Source: CAD feature listing. Evaluate the final solid. Frame: model axes, mm. Face numbers are marked on the shaded views. Coordinates: 2 decimals unless noted, no trailing zeros. Loops run counter-clockwise (first coordinate to the right, second up) from the corner with the lowest first, then second, coordinate; pieces in that order, holes last. Notation, with made-up numbers: M 2.25,3.25 L 20.25,3.25 A26 cw 20.25,42.25 Z; hole C -33,-2 d6. An arc over 180 degrees is marked long. One line per question, with ' | ' between items. Start each with the question number.
1. Mould query, pull axis Z, two halves, no side actions, for the marked faces 1, 2, 3 and 4. Classes: pulls with the +Z half, pulls with the -Z half, needs draft (parallel to the pull), parting line crosses it, or undercut.
2. Ray query, probe 1 along Y at (x, z) = (0, 0); probe 2 along Y at (x, z) = (0, 5.5); probe 3 along Z at (x, y) = (1.75, 0). Return the intervals inside material, ascending.
3. Pin query (flat end, axial travel): P1, Ø2, axis at x = 4.5, z = -0.5, coming from the -Y side; P2, Ø3, axis at y = 0, z = 0, coming from the +X side. Return the tip coordinate at first contact, or that it passes through.
4. Section query B-B, the plane z = 0. Output: boundary loops of the cut face in (x, y), and give its area (3 significant figures).
5. Section query A-A, the plane x = 0. Output: boundary loops of the cut face in (y, z), and give its area (3 significant figures).
6. Section query C-C, the plane y = -14. Output: boundary loops of the cut face in (x, z), and give its area (3 significant figures).
7. Section query D-D, the plane x = 4.75. Output: boundary loops of the cut face in (y, z), and give its area (3 significant figures).
```python
from build123d import *

# Parameters (mm, degrees)
SKETCH_R          = 1.6
PAD_DEPTH         = 6
SKETCH001_R       = 1.6
POCKET_DEPTH      = 6.001
POCKET_DEPTH_BACK = -6.001
FILLET_R          = 3


with BuildPart() as part:
    # Sketch → Pad (new body, symmetric)
    with BuildSketch(Plane.XY):
        Polygon((-6, 20), (0, 20), (6, 20), (6, 0), (6, -20), (0, -20), (-6, -20), (-6, 0), align=None)
        with Locations((0, 14)):
            Circle(SKETCH_R, mode=Mode.SUBTRACT)
        with Locations((0, -14)):
            Circle(SKETCH_R, mode=Mode.SUBTRACT)
    extrude(amount=PAD_DEPTH, both=True)

    # Sketch001 → Pocket (cut, two sides)
    with BuildSketch(Plane.YZ) as pocket_sk:
        Circle(SKETCH001_R)
    extrude(amount=-POCKET_DEPTH, mode=Mode.SUBTRACT)
    extrude(pocket_sk.sketch, amount=-POCKET_DEPTH_BACK, mode=Mode.SUBTRACT)

    # Fillet
    fillet_edges = [part.edges().sort_by_distance(p)[0] for p in [
        (6, -20, 0),
        (-6, -20, 0),
        (-6, 20, 0),
        (6, 20, 0),
    ]]
    fillet(fillet_edges, radius=FILLET_R)


solid = part.part
```
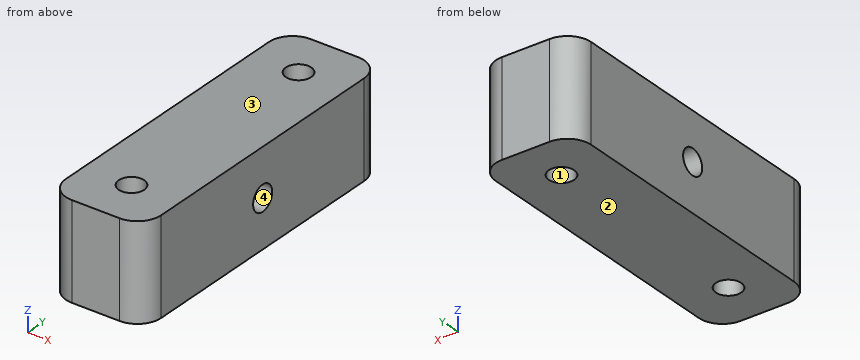
Taken from the geometry:
1) face 1: needs draft | face 2: pulls with the -Z half | face 3: pulls with the +Z half | face 4: undercut
2) probe 1: -20 to -15.6, -12.4 to -1.6, 1.6 to 12.4, 15.6 to 20 | probe 2: -20 to -15.6, -12.4 to 12.4, 15.6 to 20 | probe 3: -6 to -1.6, 1.6 to 6
3) P1: y = -19.96 | P2: through
4) outline: M -6,-17 A3 ccw -3,-20 L 3,-20 A3 ccw 6,-17 L 6,-1.6 L -6,-1.6 Z; M -6,1.6 L 6,1.6 L 6,17 A3 ccw 3,20 L -3,20 A3 ccw -6,17 Z; hole C 0,-14 d3.2; hole C 0,14 d3.2 | area: 418 mm^2
5) outline: M -20,-6 L -15.6,-6 L -15.6,6 L -20,6 Z; M -12.4,-6 L 12.4,-6 L 12.4,6 L -12.4,6 Z; M 15.6,-6 L 20,-6 L 20,6 L 15.6,6 Z; hole C 0,0 d3.2 | area: 395 mm^2
6) outline: M -6,-6 L -1.6,-6 L -1.6,6 L -6,6 Z; M 1.6,-6 L 6,-6 L 6,6 L 1.6,6 Z | area: 106 mm^2
7) outline: M -19.44,-6 L 19.44,-6 L 19.44,6 L -19.44,6 Z; hole C 0,0 d3.2 | area: 458 mm^2
